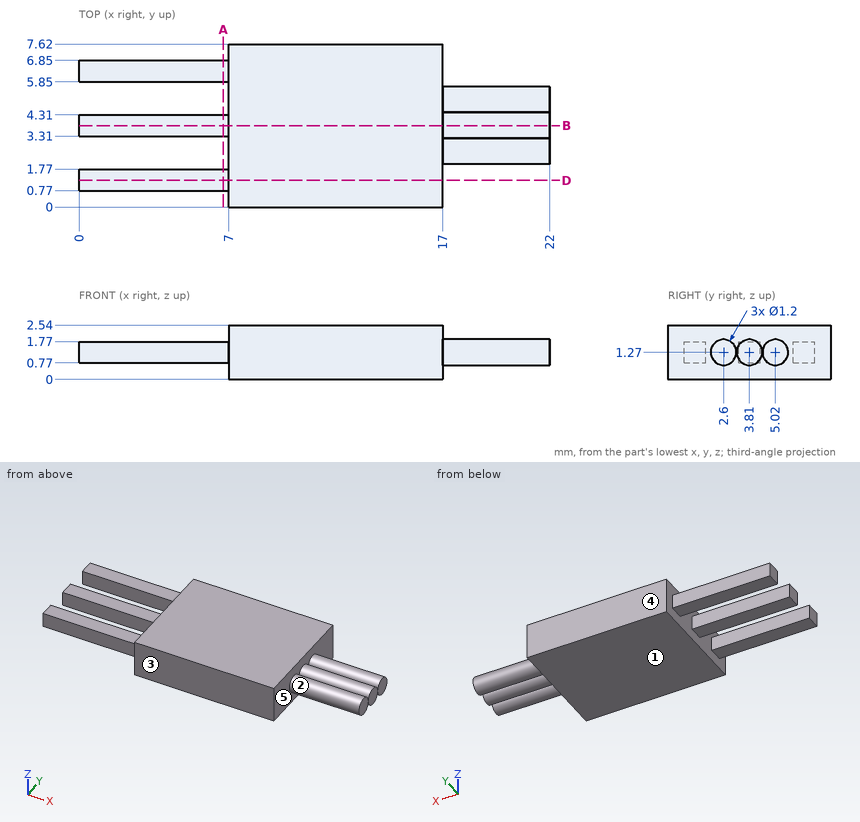
Here's the drawing with two shaded views (mm, measured from the low corner). I have some questions. A direction names the side the tool comes from. Give positions to 0.01 mm unless a question says otherwise; leave off trailing zeros. Write each loop counter-clockwise with the first axis right and the second up, starting at its lowest first coordinate (ties: lowest second). Pieces come first, ordered by that corner, then holes. Notation, with made-up numbers: (60.5, 3) -> (77.5, 3) arc R25 ccw to (77.5, 26) -> close; hole circle Ø8 at (30, 49). An arc over 180 degrees is marked (long way). Answer as a JSON object with one key per item and string values. Group by question number.
Item 1: Suppose I cut it at D-D (y = 1.25). Please give me the cut outline in (x, z).
Item 2: For the marked faces 4 and 5, which set-ups out of +Z, -Z, +X, -X, +Y, -Y let a thin tool reach every point of the face, with its end or its side?
Item 3: Suppose I cut it at B-B (y = 3.81). Please give me the cut outline in (x, z).
Item 4: Suppose I cut it at A-A (x = 6.75). Please give me the cut outline in (y, z), plus the area to 3 significant figures.
Item 5: Please list where these lines run through material, in increasing order: line 1 (Y direction, x = 2.5, z = 1.7); line 2 (X direction, y = 3, z = 1.6); line 3 (X direction, y = 5.75, z = 1.65). Write a range as [from, to].
Item 6: We'd pull the mould along Y, two halves only. Please class the marked faces 1, 2 and 3: +Y half, -Y half, draft (parallel to the pull), parting line (faces both ways), or undercut.
Item 7: I'm going to push flat-ended pins straight in: P1, Ø0.5, axis at x = 3, z = 1.5, coming from the +Y side; P2, Ø1.1, axis at x = 2.5, y = 6.5, coming from the +Z side; P3, Ø0.8, axis at x = 4, z = 1.5, coming from the -Y side. Where does each tip first touch, or does it pass through?
Findings:
{
 "1": {"outline": "(0, 0.77) -> (7, 0.77) -> (7, 0) -> (17, 0) -> (17, 2.54) -> (7, 2.54) -> (7, 1.77) -> (0, 1.77) -> close"},
 "2": {"face 4": "+Z, -Z, +X, -X, +Y", "face 5": "+X"},
 "3": {"outline": "(0, 0.77) -> (7, 0.77) -> (7, 0) -> (17, 0) -> (17, 0.67) -> (22, 0.67) -> (22, 1.87) -> (17, 1.87) -> (17, 2.54) -> (7, 2.54) -> (7, 1.77) -> (0, 1.77) -> close"},
 "4": {"outline": "(0.77, 0.77) -> (1.77, 0.77) -> (1.77, 1.77) -> (0.77, 1.77) -> close; (3.31, 0.77) -> (4.31, 0.77) -> (4.31, 1.77) -> (3.31, 1.77) -> close; (5.85, 0.77) -> (6.85, 0.77) -> (6.85, 1.77) -> (5.85, 1.77) -> close", "area": "3.00 mm²"},
 "5": {"line 1": "y = [0.77, 1.77], [3.31, 4.31], [5.85, 6.85]", "line 2": "x = [7, 22]", "line 3": "x = [7, 17]"},
 "6": {"face 1": "draft", "face 2": "undercut", "face 3": "-Y half"},
 "7": {"P1": "stops at y = 6.85", "P2": "stops at z = 1.77", "P3": "stops at y = 0.77"}
}
